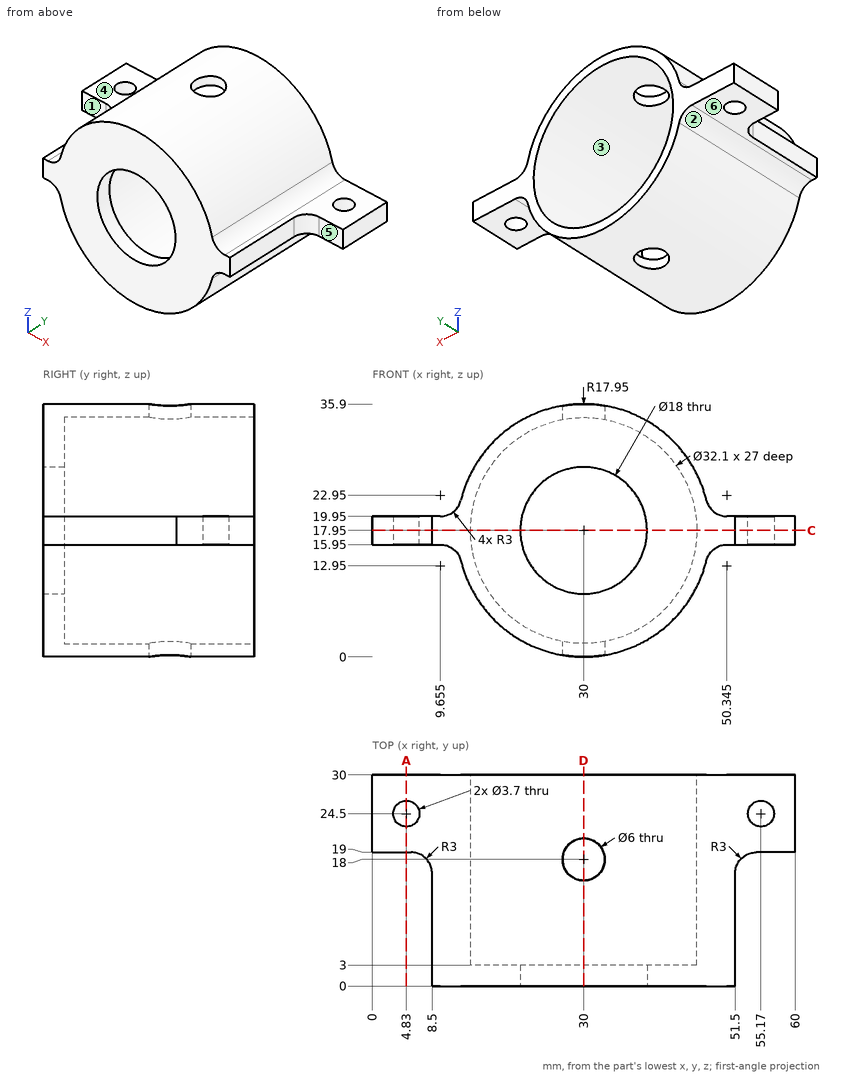
Geometry check sheet. Reference: drawing and pictorial views, mm from the part's lowest x, y, z. A direction names the side the tool comes from. Round coordinates to 2 decimals unless told otherwise and drop trailing zeros. Write each loop counter-clockwise with the first axis right and the second up, starting at its lowest first coordinate (ties: lowest second). Pieces come first, ordered by that corner, then holes.
(1) Material ranges on line 1 (Y direction, x = 55, z = 17); line 2 (Z direction, x = 30, y = 22.75); line 3 (Y direction, x = 30, z = 34.35), recorded low to high.
Returned:
line 1: y = 19 to 22.66, 26.34 to 30
line 2: z = 0 to 1.9, 34 to 35.9
line 3: y = 0 to 15, 21 to 30
(2) Section check A-A (x = 4.83). Enter the section's corners in (y, z).
Returned:
outline: (19, 15.95) - (22.65, 15.95) - (22.65, 19.95) - (19, 19.95) - close; (26.35, 15.95) - (30, 15.95) - (30, 19.95) - (26.35, 19.95) - close
(3) Access from +Z, -Z, +X, -X, +Y, -Y to the whole of each face (thin tool, end or side, straight path). Record for the marked faces 4, 5 and 6.
Returned:
face 4: +Z, -X, +Y, -Y
face 5: +Z, -Z, +X, -Y
face 6: -Z, -X, +Y, -Y
(4) Depth check by flat-ended pin: pin 1 Ø2 at (y, z) = (7.5, 17) entering from +X; pin 2 Ø5 at (x, y) = (7, 8) entering from +Z; pin 3 Ø6 at (y, z) = (14.5, 4) entering from -X; pin 4 Ø10.5 at (x, y) = (3, 9.5) entering from +Z. Enter the tip coordinate at first touch or a pass-through.
Returned:
pin 1: stops at x = 51.5
pin 2: stops at z = 19.95
pin 3: stops at x = 15.78
pin 4: passes through
(5) Section check D-D (x = 30). Enter the section's corners in (y, z).
Returned:
outline: (0, 0) - (15, 0) - (15, 1.9) - (3, 1.9) - (3, 8.95) - (0, 8.95) - close; (0, 26.95) - (3, 26.95) - (3, 34) - (15, 34) - (15, 35.9) - (0, 35.9) - close; (21, 0) - (30, 0) - (30, 1.9) - (21, 1.9) - close; (21, 34) - (30, 34) - (30, 35.9) - (21, 35.9) - close
(6) Mould release check, pull along Z, two halves, no side actions. Record for the marked faces 1, 2 and 3: pulls with the +Z half, pulls with the -Z half, needs draft (parallel to the pull), parting line crosses it, or undercut.
Returned:
face 1: needs draft
face 2: pulls with the -Z half
face 3: undercut
(7) Section check C-C (z = 17.95). Enter the section's corners in (x, y).
Returned:
outline: (0, 19) - (5.5, 19) arc R3 cw to (8.5, 16) - (8.5, 0) - (21, 0) - (21, 3) - (13.95, 3) - (13.95, 30) - (0, 30) - close; (39, 0) - (51.5, 0) - (51.5, 16) arc R3 cw to (54.5, 19) - (60, 19) - (60, 30) - (46.05, 30) - (46.05, 3) - (39, 3) - close; hole circle Ø3.7 at (4.83, 24.5); hole circle Ø3.7 at (55.17, 24.5)
